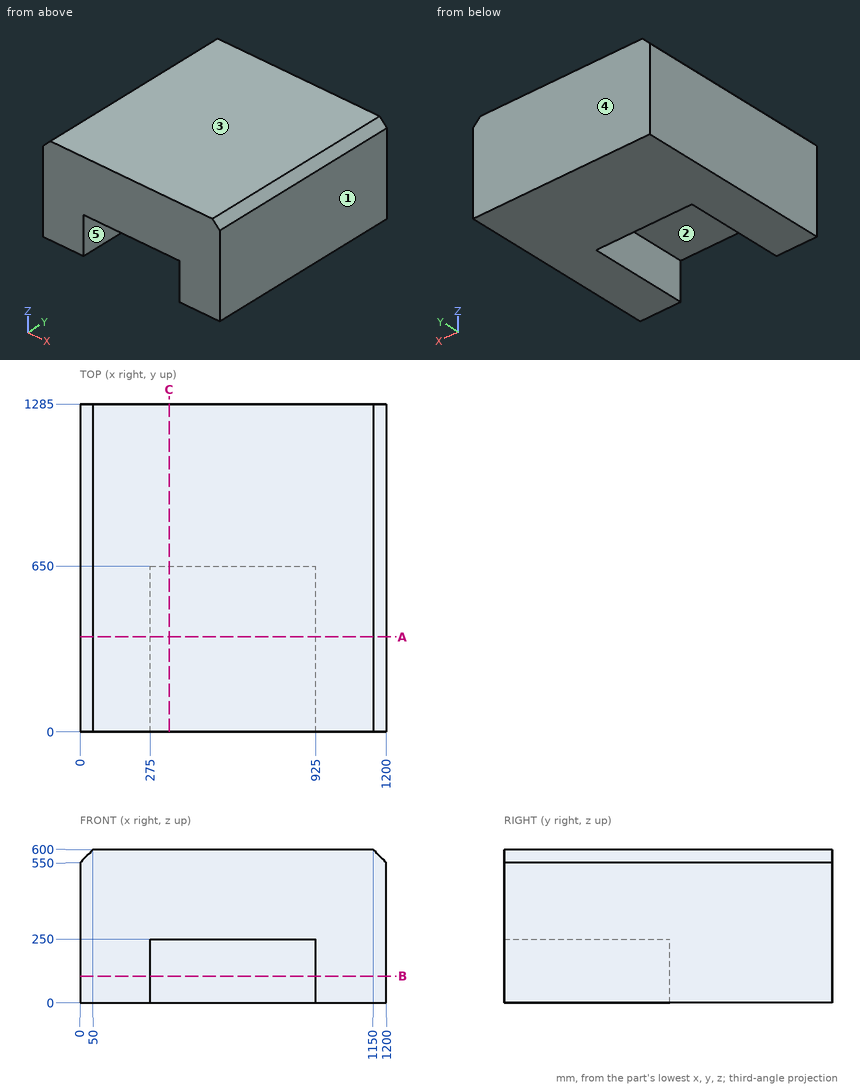
Drawing for the job (mm, zero at the part's lowest x, y, z). A direction names the side the tool comes from. Give positions to 0.01 mm unless a question says otherwise; leave off trailing zeros. Loops run counter-clockwise (first coordinate to the right, second up) from the corner with the lowest first, then second, coordinate; pieces in that order, holes last.
1) Band-saw the part on C-C on x = 349. List the corners of the cut face in (y, z), then the cut area to 4 significant figures.
Values follow:
outline: (0, 250) - (650, 250) - (650, 0) - (1285, 0) - (1285, 600) - (0, 600) - close
area: 608,500 mm2
2) Band-saw the part on A-A on y = 372.5. List the corners of the cut face in (x, z), then the cut area to 3 significant figures.
Values follow:
outline: (0, 0) - (275, 0) - (275, 250) - (925, 250) - (925, 0) - (1200, 0) - (1200, 550) - (1150, 600) - (50, 600) - (0, 550) - close
area: 555,000 mm2
3) Two-plate mould, pull along X, no slides. Class the marked faces 1, 2 and 3: released by +X, released by -X, zero draft, split by the parting line, or undercut.
Values follow:
face 1: released by +X
face 2: undercut
face 3: zero draft
4) Probe line 1 along X through (y, z) = (633.5, 199.5); line 2 along Z through (x, y) = (486, 500); line 3 along Y through (x, z) = (500.5, 128). List the from-to ranges inside material, lowest first.
Values follow:
line 1: x = 0 to 275, 925 to 1200
line 2: z = 250 to 600
line 3: y = 650 to 1285
5) 3-axis set-ups, long thin cutter, end or side, ignore diameter. For the marked faces 4 and 5: which of +Z, -Z, +X, -X, +Y, -Y reach the whole face in a straight line?
Values follow:
face 4: +Z, -Z, +X, -X, +Y
face 5: -Z, -Y
6) Band-saw the part on B-B on z = 105.5. List the corners of the cut face in (x, y), then the cut area to 3 significant figures.
Values follow:
outline: (0, 0) - (275, 0) - (275, 650) - (925, 650) - (925, 0) - (1200, 0) - (1200, 1285) - (0, 1285) - close
area: 1,120,000 mm2
7) Drop a flat-ended pin along its axis: P1, Ø1, axis at x = 644, y = 531.5, coming from the -Z side. Give the stop position or say it passes through.
Values follow:
P1: stops at z = 250
